```python
from build123d import *

# Parameters (mm, degrees)
LPATTERN1_COUNT              = 4
LPATTERN1_PITCH              = 6.0452
BOSS_EXTRUDE1_DEPTH          = 25.4
CUT_EXTRUDE1_START           = -0.635
SKETCH5_OUTSIDE_W            = 179.522
SKETCH5_OUTSIDE_H            = 184.188
SKETCH5_OUTSIDE_R            = 15.08125
CUT_EXTRUDE1_DEPTH           = 38.369131087
CUT_EXTRUDE1_TAPER           = 60
CUT_EXTRUDE1_OTHER_WAY_DEPTH = 0.635
CUT_EXTRUDE2_START           = -0.635
SKETCH6_OUTSIDE_W            = 256.438
SKETCH6_OUTSIDE_H            = 261.104
SKETCH6_OUTSIDE_R            = 15.08125
CUT_EXTRUDE2_DEPTH           = 60.572597358
CUT_EXTRUDE2_TAPER           = 60
CUT_EXTRUDE2_OTHER_WAY_DEPTH = 0.635
SKETCH7_W                    = 55.626
SKETCH7_H                    = 7.9375
FILLET1_R                    = 0.127


with BuildPart() as part:
    # Sketch2 → Revolve1 (revolve)
    with BuildSketch(Plane(origin=(0, 0, 0), x_dir=(0, 0, -1), z_dir=(1, 0, 0)), mode=Mode.PRIVATE) as revolve1_sk:
        Polygon((-30.226, 9.525), (-6.0452, 9.525), (0, 10.0965), (0, 0), (-30.226, 0), align=None)
    revolve(revolve1_sk.sketch.rotate(Axis((0, 0, 30.226), (0, 0, -1)), 180), axis=Axis((0, 0, 30.226), (0, 0, -1)))

    # Sketch3 → Revolve2 (revolve)
    with BuildSketch(Plane(origin=(0, 0, 0), x_dir=(0, 0, -1), z_dir=(1, 0, 0)), mode=Mode.PRIVATE) as revolve2_sk:
        Polygon((-30.226, 9.525), (-24.1808, 10.0965), (-24.1808, 9.525), align=None)
    revolve2 = revolve(revolve2_sk.sketch.rotate(Axis((0, 0, 0), (0, 0, 1)), 180), axis=Axis((0, 0, 0), (0, 0, 1)))

    # LPattern1: Revolve2 ×4
    with Locations(*[(0, 0, -i * LPATTERN1_PITCH) for i in range(1, LPATTERN1_COUNT)]):
        add(revolve2)

    # Sketch4 → Boss-Extrude1 (add)
    with BuildSketch(Plane(origin=(0, 0, 0), x_dir=(-1, 0, 0), z_dir=(0, 0, -1))):
        Polygon((0, 17.414327494), (-15.08125, 8.707163747), (-15.08125, -8.707163747), (0, -17.414327494), (15.08125, -8.707163747), (15.08125, 8.707163747), align=None)
    extrude(amount=BOSS_EXTRUDE1_DEPTH)

    # Sketch5 outside → Cut-Extrude1 (cut)
    with BuildSketch(Plane.XY.offset(CUT_EXTRUDE1_START)):
        Rectangle(SKETCH5_OUTSIDE_W, SKETCH5_OUTSIDE_H)
        Circle(SKETCH5_OUTSIDE_R, mode=Mode.SUBTRACT)
    extrude(amount=-CUT_EXTRUDE1_DEPTH, taper=CUT_EXTRUDE1_TAPER, mode=Mode.SUBTRACT)

    # Sketch5 outside → Cut-Extrude1 other way (cut)
    with BuildSketch(Plane.XY.offset(CUT_EXTRUDE1_START)):
        Rectangle(SKETCH5_OUTSIDE_W, SKETCH5_OUTSIDE_H)
        Circle(SKETCH5_OUTSIDE_R, mode=Mode.SUBTRACT)
    extrude(amount=CUT_EXTRUDE1_OTHER_WAY_DEPTH, mode=Mode.SUBTRACT)

    # Sketch6 outside → Cut-Extrude2 (cut)
    with BuildSketch(Plane(origin=(0, 0, -25.4), x_dir=(-1, 0, 0), z_dir=(0, 0, -1)).offset(CUT_EXTRUDE2_START)):
        Rectangle(SKETCH6_OUTSIDE_W, SKETCH6_OUTSIDE_H)
        with Locations(Location((0, 0, 0), (0, 0, 180))):
            Circle(SKETCH6_OUTSIDE_R, mode=Mode.SUBTRACT)
    extrude(amount=-CUT_EXTRUDE2_DEPTH, taper=CUT_EXTRUDE2_TAPER, mode=Mode.SUBTRACT)

    # Sketch6 outside → Cut-Extrude2 other way (cut)
    with BuildSketch(Plane(origin=(0, 0, -25.4), x_dir=(-1, 0, 0), z_dir=(0, 0, -1)).offset(CUT_EXTRUDE2_START)):
        Rectangle(SKETCH6_OUTSIDE_W, SKETCH6_OUTSIDE_H)
        with Locations(Location((0, 0, 0), (0, 0, 180))):
            Circle(SKETCH6_OUTSIDE_R, mode=Mode.SUBTRACT)
    extrude(amount=CUT_EXTRUDE2_OTHER_WAY_DEPTH, mode=Mode.SUBTRACT)

    # Sketch7 → Cut-Revolve1 (revolve, cut)
    with BuildSketch(Plane(origin=(0, 0, 0), x_dir=(0, 0, -1), z_dir=(1, 0, 0)), mode=Mode.PRIVATE) as cut_revolve1_sk:
        with Locations((-2.413, 3.96875)):
            Rectangle(SKETCH7_W, SKETCH7_H)
    revolve(cut_revolve1_sk.sketch.rotate(Axis((0, 0, 30.226), (0, 0, -1)), 270), axis=Axis((0, 0, 30.226), (0, 0, -1)), mode=Mode.SUBTRACT)

    # Sketch8 → Cut-Revolve2 (revolve, cut)
    with BuildSketch(Plane(origin=(0, 0, 0), x_dir=(0, 0, -1), z_dir=(1, 0, 0)), mode=Mode.PRIVATE) as cut_revolve2_sk:
        Polygon((25.4, 13.335), (11.53922, 12.903443324), (11.53922, 11.7078125), (4.504456534, 0), (25.4, 0), align=None)
    revolve(cut_revolve2_sk.sketch.rotate(Axis((0, 0, 30.226), (0, 0, -1)), 270), axis=Axis((0, 0, 30.226), (0, 0, -1)), mode=Mode.SUBTRACT)

    # Fillet1
    fillet1_edges = [part.edges().sort_by_distance(p)[0] for p in [
        (0, 9.525, 30.226),
        (0, 10.0965, 0),
    ]]
    fillet(fillet1_edges, radius=FILLET1_R)


solid = part.part
```
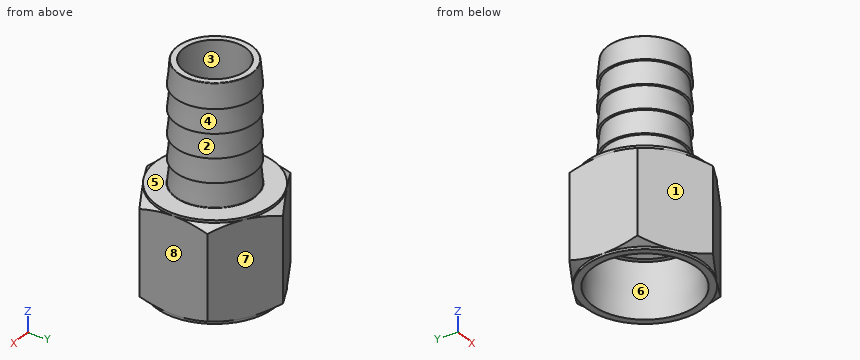
Design review of the part built by this model. Coordinates are the model's own, in mm. Face numbers are marked on the shaded views. A direction names the side the tool comes from. Give positions to 0.01 mm unless a question says otherwise; leave off trailing zeros. Order: outer loops, then holes, each group sorted by start corner. A loop starts at its lowest first (then second) coordinate and runs counter-clockwise, first axis right, second up. Notation, with made-up numbers: M 8.25,-33.5 L 17.25,-33.5 A8 cw 17.25,-27.5 Z; hole C 83.25,-23.5 d11. An arc over 180 degrees is marked long. One line per question, with ' | ' between items. Start each with the question number.
Q1. Machinability: for the marked faces 4, 5, 6, 7 and 8, which of the approach directions +Z, -Z, +X, -X, +Y, -Y give a long, thin tool a straight path to every point of the face, cutting with its end or side? Answer none if there is none.
Q2. For pin 1 Ø3 at (x, z) = (-7.5, -0.5) entering from +Y; pin 2 Ø13 at (x, y) = (2, -1.5) entering from -Z; pin 3 Ø5 at (y, z) = (4, 6.5) entering from -X, all flat-tipped, find the tip position at first contact; note any pin that passes through.
Q3. We need section B-B (z = 19). Write out the cut boundary in (x, y) (1 decimal), plus the area to 3 significant figures.
Q4. We need section A-A (z = -15). Write out the cut boundary in (x, y), plus the area to 3 significant figures.
Q5. For L1, parallel to Z at x = -0.5, y = -12.5; L2, parallel to Y at x = 0, z = 11; L3, parallel to X at y = 0, z = 9.5, list the stretches that pass through material, from the lowest coordinate up. Write a range as [from, to].
Q6. The part is to be moulded in two halves that separate along X. For the marked faces 1, 2 and 3, say which applies: +X half, -X half, draft (parallel to the pull), parting line (faces both ways), or undercut.
Q7. We need section C-C (z = 26). Write out the cut boundary in (x, y) (1 decimal), plus the area to 3 significant figures.
Returned:
1) face 4: none | face 5: +Z | face 6: -Z | face 7: +Z, -Z, +X, +Y | face 8: +Z, -Z, +X, +Y, -Y
2) pin 1: y = 13.94 | pin 2: z = -9.91 | pin 3: x = -9.98
3) outline: C 0,0 d20; hole C 0,0 d15.9 | area: 117 mm2
4) outline: M -15.08,-8.71 L 0,-17.41 L 15.08,-8.71 L 15.08,8.71 L 0,17.41 L -15.08,8.71 Z; hole C 0,0 d26.02 | area: 256 mm2
5) L1: [-11.54, 0] | L2: [-9.63, -7.94], [7.94, 9.63] | L3: [-9.77, -7.94], [7.94, 9.77]
6) face 1: -X half | face 2: parting line | face 3: undercut
7) outline: C 0,0 d19.8; hole C 0,0 d15.9 | area: 112 mm2
